Verification items for the finished model (mm, model axes). A direction names the side the tool comes from. Round coordinates to 2 decimals unless told otherwise and drop trailing zeros. Write each loop counter-clockwise with the first axis right and the second up, starting at its lowest first coordinate (ties: lowest second). Pieces come first, ordered by that corner, then holes. Notation, with made-up numbers: (45, 86) - (53, 86) arc R15 ccw to (53, 104) - close; hole circle Ø9 at (69.25, 2). An arc over 180 degrees is marked (long way). Answer as a JSON object with one key per item and string values. Group by question number.
1) Mould release check, pull along X, two halves, no side actions. Record for faces 1 (the cylindrical face through (13.17, -77.92, 8.95)), 2 (the cylindrical face through (-10.805, -165.975, 8.96)), 3 (the flat face through (3.549, -138.974, 9.122)): +X half, -X half, draft (parallel to the pull), parting line (faces both ways), or undercut.
2) Set-up check for faces 4 (the cylindrical face through (-13.17, -77.92, 8.95)), 5 (the flat face through (-3.2, -89.34, 5.67)): record each of +Z, -Z, +X, -X, +Y, -Y from which the full face is reachable in a straight line by a thin tool's end or side.
3) Go/stop test with flat-tipped pins: pin 1 Ø4 at (x, y) = (-2.5, -96.5) entering from +Z; pin 2 Ø10.5 at (x, y) = (1.5, -20.5) entering from +Z; pin 3 Ø4 at (y, z) = (-121, 5.5) entering from -X. Record where each tip stops, or that it passes through.
4) Section check A-A (y = -70). Enter the section's corners in (x, z).
5) Section check B-B (y = -131). Enter the section's corners in (x, z).
6) Thickness scan on line 1 (X direction, y = -77, z = 1.25); line 2 (X direction, y = -143, z = 8.25); line 3 (Z direction, x = 4.5, y = -69). Record the ranges inside material, lowest first.
```python
from build123d import *

# Parameters (mm, degrees)
F1_DEPTH   = 175
F2_R       = 4.5
F3_DEPTH   = 7
F4_DEPTH   = 25
F5_SIZE2   = 1.7320508076
F5_SIZE    = 1
F6_SIZE2   = 3.5265396142
F6_SIZE    = 20
F6_2_SIZE2 = 3.5265396142
F6_2_SIZE  = 20
F7_R       = 15
F8_R       = 2


with BuildPart() as f1:
    # F0 (on Front) → F1 (new body)
    with BuildSketch(Plane.XZ):
        Polygon((-15.2520753821, 10), (-8.25, 0), (8.25, 0), (15.2520753821, 10), align=None)
    extrude(amount=F1_DEPTH)

    # F2 (on face) → F3 (cut)
    with BuildSketch(Plane.XY.offset(10)):
        Polygon((6.5, -23.7527767497), (6.5, -16.2472232503), (0, -12.4944465005), (-6.5, -16.2472232503), (-6.5, -23.7527767497), (0, -27.5055534995), align=None)
        with Locations((0, -20)):
            Circle(F2_R, mode=Mode.SUBTRACT)
        Polygon((-6.5, -41.2472232503), (-6.5, -48.7527767497), (0, -52.5055534995), (6.5, -48.7527767497), (6.5, -41.2472232503), (0, -37.4944465005), align=None)
        with Locations((0, -45)):
            Circle(F2_R, mode=Mode.SUBTRACT)
        Polygon((-6.5, -66.2472232503), (-6.5, -73.7527767497), (0, -77.5055534995), (6.5, -73.7527767497), (6.5, -66.2472232503), (0, -62.4944465005), align=None)
        with Locations((0, -70)):
            Circle(F2_R, mode=Mode.SUBTRACT)
        Polygon((-6.5, -91.2472232503), (-6.5, -98.7527767497), (0, -102.5055534995), (6.5, -98.7527767497), (6.5, -91.2472232503), (0, -87.4944465005), align=None)
        with Locations((0, -95)):
            Circle(F2_R, mode=Mode.SUBTRACT)
        Polygon((-6.5, -116.2472232503), (-6.5, -123.7527767497), (0, -127.5055534995), (6.5, -123.7527767497), (6.5, -116.2472232503), (0, -112.4944465005), align=None)
        with Locations((0, -120)):
            Circle(F2_R, mode=Mode.SUBTRACT)
        Polygon((-6.5, -141.2472232503), (-6.5, -148.7527767497), (0, -152.5055534995), (6.5, -148.7527767497), (6.5, -141.2472232503), (0, -137.4944465005), align=None)
        with Locations((0, -145)):
            Circle(F2_R, mode=Mode.SUBTRACT)
    extrude(amount=-F3_DEPTH, mode=Mode.SUBTRACT)

    # F4 (cut): faces of the model
    f4_faces = [f1.faces().sort_by_distance(p)[0] for p in [
        (0, -20, 10),
        (0, -45, 10),
        (0, -70, 10),
        (0, -95, 10),
        (0, -120, 10),
        (0, -145, 10),
    ]]
    extrude(f4_faces, amount=-F4_DEPTH, mode=Mode.SUBTRACT)

    # F5
    f5_edges = [f1.edges().sort_by_distance(p)[0] for p in [
        (-6.5, -145, 10),
        (-3.25, -139.370835, 10),
        (-3.25, -150.629165, 10),
        (3.25, -150.629165, 10),
        (6.5, -145, 10),
        (3.25, -139.370835, 10),
        (-3.25, -125.629165, 10),
        (-6.5, -120, 10),
        (-3.25, -114.370835, 10),
        (3.25, -114.370835, 10),
        (6.5, -120, 10),
        (3.25, -125.629165, 10),
        (-6.5, -95, 10),
        (-3.25, -89.370835, 10),
        (3.25, -89.370835, 10),
        (6.5, -95, 10),
        (3.25, -100.629165, 10),
        (-3.25, -100.629165, 10),
        (-3.25, -75.629165, 10),
        (-6.5, -70, 10),
        (-3.25, -64.370835, 10),
        (3.25, -64.370835, 10),
        (6.5, -70, 10),
        (3.25, -75.629165, 10),
        (-6.5, -45, 10),
        (-3.25, -39.370835, 10),
        (3.25, -39.370835, 10),
        (6.5, -45, 10),
        (3.25, -50.629165, 10),
        (-3.25, -50.629165, 10),
        (-3.25, -25.629165, 10),
        (-6.5, -20, 10),
        (-3.25, -14.370835, 10),
        (3.25, -14.370835, 10),
        (6.5, -20, 10),
        (3.25, -25.629165, 10),
    ]]
    chamfer(f5_edges, length=F5_SIZE, length2=F5_SIZE2)

    # F6
    f6_edges = [f1.edges().sort_by_distance(p)[0] for p in [
        (-11.751038, -175, 5),
    ]]
    f6_side = f1.faces().sort_by_distance((-11.751038, -87.5, 5))[0]
    chamfer(f6_edges, length=F6_SIZE, length2=F6_SIZE2, reference=f6_side)

    # F6#2
    f6_2_edges = [f1.edges().sort_by_distance(p)[0] for p in [
        (11.751038, -175, 5),
    ]]
    f6_2_side = f1.faces().sort_by_distance((11.751038, -87.5, 5))[0]
    chamfer(f6_2_edges, length=F6_2_SIZE, length2=F6_2_SIZE2, reference=f6_2_side)

    # F7
    f7_edges = [f1.edges().sort_by_distance(p)[0] for p in [
        (-11.751038, -155, 5),
        (11.751038, -155, 5),
    ]]
    fillet(f7_edges, radius=F7_R)

    # F8
    f8_edges = [f1.edges().sort_by_distance(p)[0] for p in [
        (12.960423, -165.646196, 10),
        (-12.960423, -165.646196, 10),
    ]]
    fillet(f8_edges, radius=F8_R)


solid = f1.part
```
Returned:
{
 "1": {"face 1": "+X half", "face 2": "-X half", "face 3": "undercut"},
 "2": {"face 4": "-X, +Y, -Y", "face 5": "+Z"},
 "3": {"pin 1": "z = 3", "pin 2": "z = 8.7", "pin 3": "x = -13.35"},
 "4": {"outline": "(-13.05, 6.85) - (-8.25, 0) - (-4.5, 0) - (-4.5, 3) - (-6.5, 3) - (-6.5, 8.27) - (-7.5, 10) - (-11.41, 10) arc R2 ccw to start; (4.5, 0) - (8.25, 0) - (13.05, 6.85) arc R2 ccw to (11.41, 10) - (7.5, 10) - (6.5, 8.27) - (6.5, 3) - (4.5, 3) - close"},
 "5": {"outline": "(-13.05, 6.85) - (-8.25, 0) - (8.25, 0) - (13.05, 6.85) arc R2 ccw to (11.41, 10) - (-11.41, 10) arc R2 ccw to start"},
 "6": {"line 1": "-9.13 to 9.13", "line 2": "-13.39 to -6.5, 6.5 to 13.39", "line 3": "0 to 3"}
}
